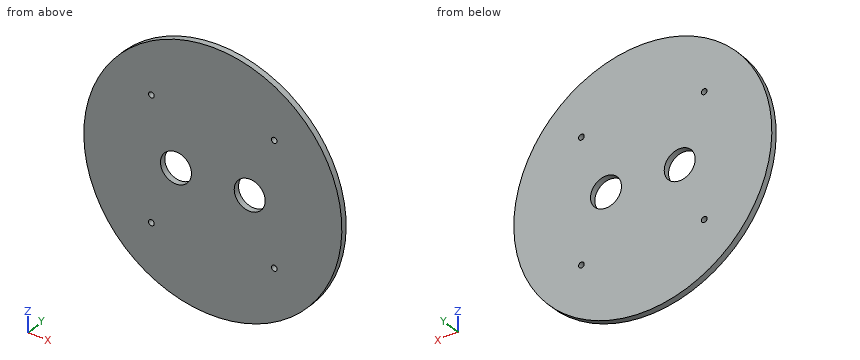
from build123d import *

# Parameters (mm, degrees)
SKETCH1_R             = 66.675
BOSS_EXTRUDE1_DEPTH   = 3.175
HOLE1_D               = 16.002
F_4_CLEARANCE_HOLE1_D = 2.9464
LPATTERN1_COUNT       = 2
LPATTERN1_PITCH       = 63.5
LPATTERN1_COUNT_DIR2  = 2
LPATTERN1_PITCH_DIR2  = 63.5


with BuildPart() as part:
    # Sketch1 → Boss-Extrude1 (new body)
    with BuildSketch(Plane(origin=(0, 0, 0), x_dir=(1, 0, 0), z_dir=(0, 1, 0))):
        with Locations(Location((0, 0, 0), (0, 0, 270))):
            Circle(SKETCH1_R)
    extrude(amount=BOSS_EXTRUDE1_DEPTH)

    # Hole1 (through all)
    with Locations(Plane(origin=(0, 3.175, 0), x_dir=(1, 0, 0), z_dir=(0, 1, 0))):
        with Locations((19.05, 0)):
            hole1 = Hole(HOLE1_D / 2)

    # Mirror1: Hole1 across plane
    add(hole1.mirror(Plane(origin=(0, 0, 0), x_dir=(0, 0, 1), z_dir=(1, 0, 0))), mode=Mode.SUBTRACT)

    # #4 Clearance Hole1 (through all)
    with Locations(Plane(origin=(0, 3.175, 0), x_dir=(1, 0, 0), z_dir=(0, 1, 0))):
        with Locations((-31.75, 31.75)):
            f_4_clearance_hole1 = Hole(F_4_CLEARANCE_HOLE1_D / 2)

    # LPattern1: 4 Clearance Hole1 2 × 2
    with Locations(*[(i * LPATTERN1_PITCH, 0, j * LPATTERN1_PITCH_DIR2) for i in range(LPATTERN1_COUNT) for j in range(LPATTERN1_COUNT_DIR2) if (i, j) != (0, 0)]):
        add(f_4_clearance_hole1, mode=Mode.SUBTRACT)


solid = part.part
Build history of the part. All positions in model axes, mm. Give positions to 0.01 mm unless a question says otherwise; leave off trailing zeros. Loops run counter-clockwise (first coordinate to the right, second up) from the corner with the lowest first, then second, coordinate; pieces in that order, holes last. Notation, with made-up numbers: (-1, -40) -> (52, -40) arc R15 ccw to (52, -21) -> close; hole circle Ø1 at (-2, 89). An arc over 180 degrees is marked (long way). Answer in a Markdown table with one row per item.
Item 1: Slice it at C-C on x = 16. Write the cut outline in (y, z) (3 decimals).
Findings below:
| item | result |
|---|---|
| outline | (0, -64.727) -> (3.175, -64.727) -> (3.175, -7.397) -> (0, -7.397) -> close; (0, 7.397) -> (3.175, 7.397) -> (3.175, 64.727) -> (0, 64.727) -> close |
Item 2: Slice it at A-A on y = 0.7. Write the cut outline in (x, z) (3 decimals), plus the area to 3 significant figures.
Findings below:
| item | result |
|---|---|
| outline | circle Ø133.35 at (0, 0); hole circle Ø2.946 at (-31.75, -31.75); hole circle Ø2.946 at (-31.75, 31.75); hole circle Ø16.002 at (-19.05, 0); hole circle Ø16.002 at (19.05, 0); hole circle Ø2.946 at (31.75, -31.75); hole circle Ø2.946 at (31.75, 31.75) |
| area | 13,500 mm² |
Item 3: Flat gauge pin, fed straight in: P1, Ø2.5, axis at x = 31.75, z = 31.75, coming from the -Y side. Where does the tip first touch, or does it go through?
Findings below:
| item | result |
|---|---|
| P1 | passes through |
Item 4: Probe line 1 along Z through (x, y) = (31.75, 1.05); line 2 along X through (y, z) = (0.25, 1.5). List the from-to ranges inside material, lowest first. Write a range as [from, to].
Findings below:
| item | result |
|---|---|
| line 1 | z = [-58.63, -33.22], [-30.28, 30.28], [33.22, 58.63] |
| line 2 | x = [-66.66, -26.91], [-11.19, 11.19], [26.91, 66.66] |
Item 5: Slice it at B-B on z = 0. Write the cut outline in (x, y) (3 decimals).
Findings below:
| item | result |
|---|---|
| outline | (-66.675, 0) -> (-27.051, 0) -> (-27.051, 3.175) -> (-66.675, 3.175) -> close; (-11.049, 0) -> (11.049, 0) -> (11.049, 3.175) -> (-11.049, 3.175) -> close; (27.051, 0) -> (66.675, 0) -> (66.675, 3.175) -> (27.051, 3.175) -> close |
Item 6: Slice it at D-D on x = -19.05. Write the cut outline in (y, z) (3 decimals).
Findings below:
| item | result |
|---|---|
| outline | (0, -63.896) -> (3.175, -63.896) -> (3.175, -8.001) -> (0, -8.001) -> close; (0, 8.001) -> (3.175, 8.001) -> (3.175, 63.896) -> (0, 63.896) -> close |
